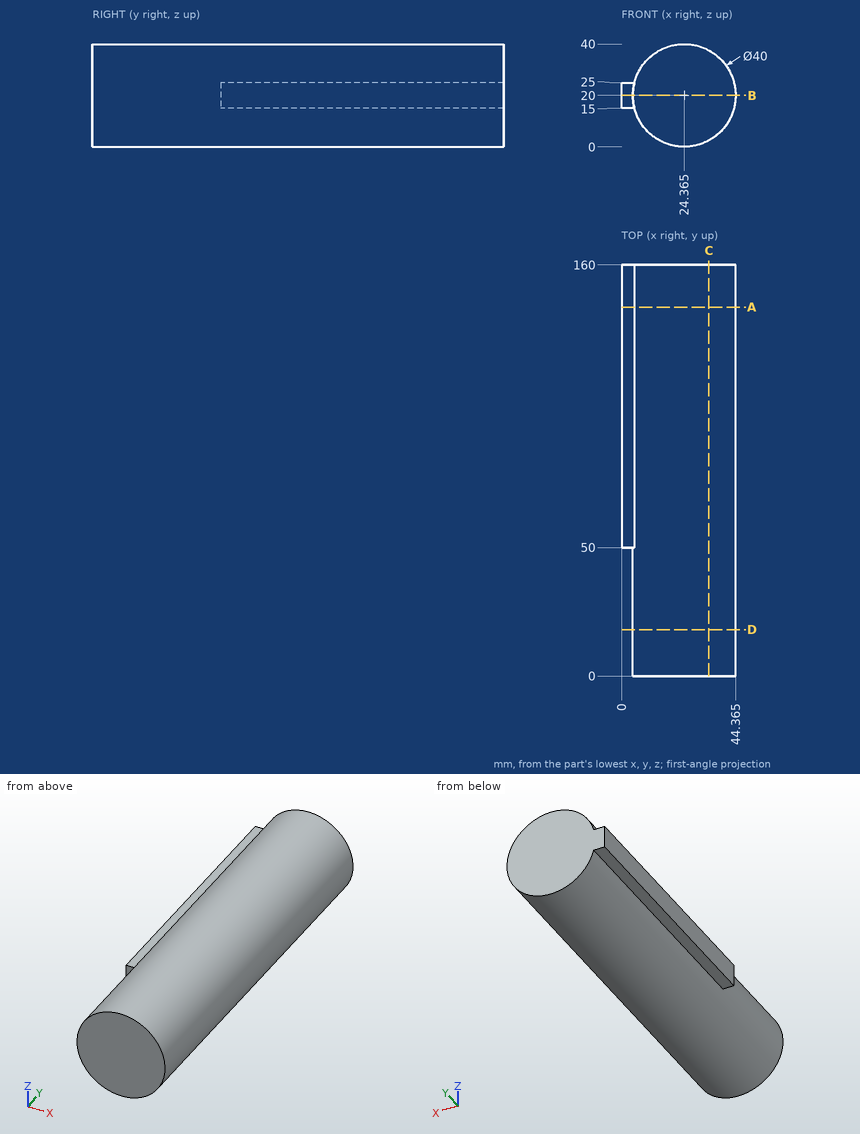
Study the drawing (mm; zero at the part's minimum x, y, z) and answer. Round coordinates to 2 decimals unless told otherwise and drop trailing zeros. Loops run counter-clockwise (first coordinate to the right, second up) from the corner with the lowest first, then second, coordinate; pieces in that order, holes last. Notation, with made-up numbers: M 76.5,51.5 L 97.5,51.5 A25 ccw 97.5,77.5 Z; hole C -11.5,54.5 d11. An arc over 180 degrees is marked long. One line per question, with ' | ' between items.
Q1. Find section D-D, the plane y = 18. Give the vertices of the cut face in (x, z) (3 decimals), then the cut area to 3 significant figures.
Conclusion:
outline: C 24.365,20 d40 | area: 1,260 mm2
Q2. Find section B-B, the plane z = 20. Give the vertices of the cut face in (x, y) (3 decimals), then the cut area to 3 significant figures.
Conclusion:
outline: M 0,50 L 4.365,50 L 4.365,0 L 44.365,0 L 44.365,160 L 0,160 Z | area: 6,880 mm2
Q3. Consider line 1 along X through (y, z) = (15, 20) (3 decimals); line 2 along Z through (x, y) = (42, 136) (1 decimal); line 3 along Z through (x, y) = (40, 124). Determine where each line is inside the solid, lowest interval first. Write a range as from..to.
Conclusion:
line 1: x = 4.365..44.365 | line 2: z = 10.6..29.4 | line 3: z = 7.53..32.47
Q4. Find section A-A, the plane y = 143.5. Give the vertices of the cut face in (x, z) (3 decimals).
Conclusion:
outline: M 0,15 L 5,15 A20 ccw long 5,25 L 0,25 Z
Q5. Each of these flat-tipped pins is pushed along its axis until it touches: pin 1 Ø2.5 at (x, y) = (1.5, 79.5) entering from +Z; pin 2 Ø10 at (y, z) = (29, 6.5) entering from -X; pin 3 Ø12 at (y, z) = (54.5, 16.5) entering from +X (3 decimals). Where does it stop, or does it pass through?
Conclusion:
pin 1: stops at z = 25 | pin 2: stops at x = 6.26 | pin 3: stops at x = 44.365
Q6. Find section C-C, the plane x = 34. Give the vertices of the cut face in (y, z).
Conclusion:
outline: M 0,2.47 L 160,2.47 L 160,37.53 L 0,37.53 Z
